from build123d import *

# Parameters (mm, degrees)
SKETCH_1_R          = 12.5
SKETCH_1_R_2        = 5
EXTRUDE_1_DEPTH     = 40
SKETCH_9_W          = 9.82849153
SKETCH_9_H          = 17.418402746
EXTRUDE_4_DEPTH     = 15
SKETCH_12_R         = 2.492986731
CUT_EXTRUDE_2_DEPTH = 65.854299957
CUT_EXTRUDE_3_DEPTH = 65.854299957
CUT_EXTRUDE_4_DEPTH = 65.854299957
CUT_EXTRUDE_5_DEPTH = 15


with BuildPart() as part:
    # Sketch 1 → Extrude 1 (new body)
    with BuildSketch(Plane(origin=(0, 0, 0), x_dir=(1, 0, 0), z_dir=(0, 1, 0))):
        with Locations(Location((0, 0, 0), (0, 0, 270))):
            Circle(SKETCH_1_R)
        with Locations(Location((0, 0, 0), (0, 0, 270))):
            Circle(SKETCH_1_R_2, mode=Mode.SUBTRACT)
    extrude(amount=EXTRUDE_1_DEPTH)

    # Sketch 4 → Revolve 2 (revolve)
    with BuildSketch(Plane(origin=(0, 0, 0), x_dir=(0, 0, -1), z_dir=(1, 0, 0))):
        Polygon((-10, 45), (0, 45), (0, 39.999913314), (-12.5, 40), align=None)
    revolve(axis=Axis((0, 39.999913314, 0), (0, 1, 0)))

    # Sketch 9 → Extrude 4 (add)
    with BuildSketch(Plane(origin=(0, 45, 0), x_dir=(1, 0, 0), z_dir=(0, 1, 0))):
        Rectangle(SKETCH_9_W, SKETCH_9_H)
    extrude(amount=EXTRUDE_4_DEPTH)

    # Sketch 12 → Cut-Extrude 2 (cut, through all)
    with BuildSketch(Plane.XY.offset(8.709201373)):
        with Locations((0, 52)):
            Circle(SKETCH_12_R)
    extrude(amount=-CUT_EXTRUDE_2_DEPTH, mode=Mode.SUBTRACT)

    # Sketch 12_4 → Cut-Extrude 3 (cut, through all)
    with BuildSketch(Plane.XY.offset(8.709201373)):
        with BuildLine():
            Line((0, 57.060476342), (0, 60))
            Line((0, 60), (-4.914245765, 60))
            Line((-4.914245765, 60), (-4.914245765, 52.146230577))
            ThreePointArc((-4.914245765, 52.146230577), (-3.474896505, 55.621127082), (0, 57.060476342))
        make_face()
    extrude(amount=-CUT_EXTRUDE_3_DEPTH, mode=Mode.SUBTRACT)

    # Sketch 14 → Cut-Extrude 4 (cut, through all)
    with BuildSketch(Plane.XY.offset(8.709201373)):
        with BuildLine():
            ThreePointArc((-4.534941492, 54.039407036), (0.668025232, 56.927333729), (4.914245765, 52.758329712))
            Line((4.914245765, 52.758329712), (4.914245765, 53.845840784))
            Line((4.914245765, 53.845840784), (4.914245765, 60))
            Line((4.914245765, 60), (0, 60))
            Line((0, 60), (0, 57.060476342))
            ThreePointArc((0, 57.060476342), (-2.724543727, 56.236056113), (-4.534941492, 54.039407036))
        make_face()
    extrude(amount=-CUT_EXTRUDE_4_DEPTH, mode=Mode.SUBTRACT)

    # Sketch 15 → Cut-Extrude 5 (cut)
    with BuildSketch(Plane(origin=(4.914245765, 0, 0), x_dir=(0, 0, -1), z_dir=(1, 0, 0))):
        Polygon((-3, 45), (-3, 52.758329712), (-3, 60.738034658), (3, 60.738034658), (3, 45), (0, 45), align=None)
    extrude(amount=-CUT_EXTRUDE_5_DEPTH, mode=Mode.SUBTRACT)


solid = part.part
Geometry check sheet. Reference: the model listing, model coordinates, mm. A direction names the side the tool comes from. Coordinates: 2 decimals unless noted, no trailing zeros. Order: outer loops, then holes, each group sorted by start corner. A loop starts at its lowest first (then second) coordinate and runs counter-clockwise, first axis right, second up. Notation, with made-up numbers: (46, -23) - (59, -23) arc R27 cw to (59, 0) - close; hole circle Ø3 at (45, 80.25). An arc over 180 degrees is marked (long way). Answer in a Markdown table with one row per item. Add a question column.
1) Material ranges on line 1 along Y through (x, z) = (0, 6.15); line 2 along Y through (x, z) = (0, -4.15); line 3 along X through (y, z) = (25, 0), recorded low to high. Write a range as [from, to].
2) Gauge pin test, flat ends, axial feed: P1, Ø5, axis at y = 11.5, z = 4, coming from the +X side; P2, Ø3, axis at x = 1, y = 49, coming from the -Z side; P3, Ø11.5, axis at x = 0, z = 0, coming from the +Y side; P4, Ø8, axis at x = 0, y = 52, coming from the +Z side. Record the tip position at first contact, or that the pin passes through.
3) Cross-section at A-A, the plane y = 26. Record the cut outline in (x, z).
4) Release check for a two-part mould opening along X. For faces 1 (the cylindrical face through (-0.54, 49.566, -5.815)), 2 (the flat face through (4.914, 49, -6)), 3 (the flat face through (-5.4, 0, -0.2)) record: +X half, -X half, draft (parallel to the pull), parting line (faces both ways), or undercut.
5) Set-up check for faces 4 (the conical face through (0, 40, 0)), 5 (the flat face through (0, 45, 9)), 6 (the flat face through (-4.914, 49, -6)): record each of +Z, -Z, +X, -X, +Y, -Y from which the full face is reachable in a straight line by a thin tool's end or side.
Check result:
| question | item | result |
|---|---|---|
| 1 | line 1 | y = [0, 49.51], [54.49, 56.97] |
| 1 | line 2 | y = [40, 49.51], [54.49, 56.97] |
| 1 | line 3 | x = [-12.5, -5], [5, 12.5] |
| 2 | P1 | stops at x = 12.41 |
| 2 | P2 | stops at z = -8.71 |
| 2 | P3 | stops at y = 56.97 |
| 2 | P4 | stops at z = 8.71 |
| 3 | outline | circle Ø25 at (0, 0); hole circle Ø10 at (0, 0) |
| 4 | face 1 | undercut |
| 4 | face 2 | +X half |
| 4 | face 3 | draft |
| 5 | face 4 | -Y |
| 5 | face 5 | +Z, +X, -X, +Y |
| 5 | face 6 | +Z, -Z, -X, +Y |
